Drawing for the job (mm, zero at the part's lowest x, y, z). Round coordinates to 2 decimals unless told otherwise and drop trailing zeros. Write each loop counter-clockwise with the first axis right and the second up, starting at its lowest first coordinate (ties: lowest second). Pieces come first, ordered by that corner, then holes. Notation, with made-up numbers: M 9,20 L 48,20 A9 cw 48,37 Z; hole C -19,1 d4. An arc over 180 degrees is marked long. Use a Markdown table: item, result. Add a question column.
1) Drop flat-ended pins along their axis: P1, Ø1.5, axis at x = 18, z = 23.5, coming from the -Y side; P2, Ø2, axis at x = 9.5, z = 25.5, coming from the -Y side; P3, Ø1, axis at x = 9.5, z = 31.5, coming from the -Y side. Give the stop position or say it passes through.
2) Wall check: probe 1 along X at (y, z) = (30.5, 24); probe 2 along Y at (x, z) = (17, 51.5); probe 3 along Y at (x, z) = (29, 33). Give the ranges that are in metal, low to high.
3) Slice it at A-A on y = 6. Write the cut outline in (x, z), plus the area to 3 significant figures.
4) Slice it at D-D on z = 28.5. Write the cut outline in (x, y), plus the area to 3 significant figures.
5) Slice it at B-B on x = 5. Write the cut outline in (y, z).
6) Slice it at C-C on z = 22. Write the cut outline in (x, y), plus the area to 3 significant figures.
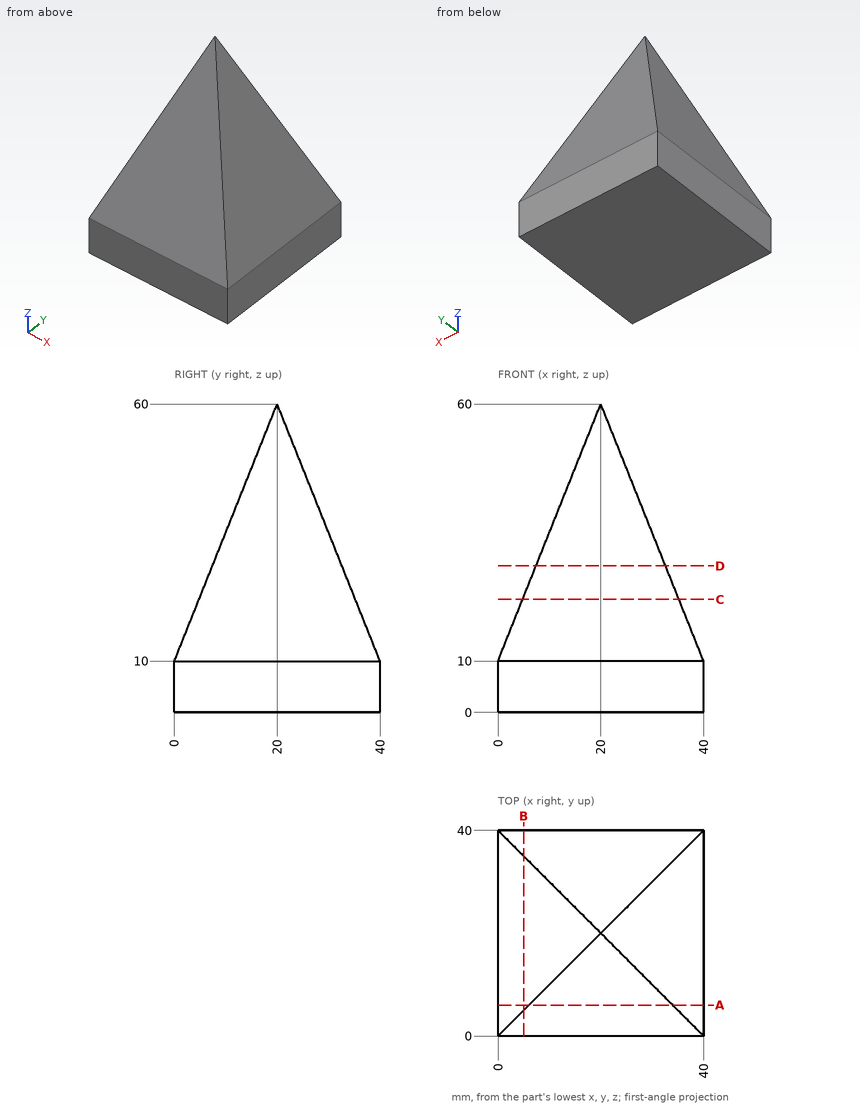
Entries:
| question | item | result |
|---|---|---|
| 1 | P1 | stops at y = 5.1 |
| 1 | P2 | stops at y = 5.8 |
| 1 | P3 | stops at y = 8.4 |
| 2 | probe 1 | x = 5.6 to 34.4 |
| 2 | probe 2 | y = 16.6 to 23.4 |
| 2 | probe 3 | y = 9.2 to 30.8 |
| 3 | outline | M 0,0 L 40,0 L 40,10 L 34,25 L 6,25 L 0,10 Z |
| 3 | area | 910 mm^2 |
| 4 | outline | M 7.4,7.4 L 32.6,7.4 L 32.6,32.6 L 7.4,32.6 Z |
| 4 | area | 635 mm^2 |
| 5 | outline | M 0,0 L 40,0 L 40,10 L 35,22.5 L 5,22.5 L 0,10 Z |
| 6 | outline | M 4.8,4.8 L 35.2,4.8 L 35.2,35.2 L 4.8,35.2 Z |
| 6 | area | 924 mm^2 |
